The listing builds one solid part. Answer for the finished solid, in the listing's coordinates (mm). A direction names the side the tool comes from. Round coordinates to 2 decimals unless told otherwise and drop trailing zeros. Write each loop counter-clockwise with the first axis right and the second up, starting at its lowest first coordinate (ties: lowest second). Pieces come first, ordered by that corner, then holes.
Item 1: For a pull along X with two mould halves and no side action, classify faces 3 (the face through (-29.289, 4.196, 5.07)), 4 (the face through (-13, -6, 5)), 5 (the face through (-14.669, 0.526, 4.93)) as +X half, -X half, draft (parallel to the pull), parting line (faces both ways), or undercut.
Item 2: Find the intervals of material crossed by probe 1 along Y at (x, z) = (-13, 3); probe 2 along Z at (x, y) = (-6, -4); probe 3 along X at (y, z) = (0.5, 108.5), in increasing order.
Item 3: Each of these flat-tipped pins is pushed along its axis until it touches: pin 1 (6 mm diameter, centred on x = -13.5, y = 2, fed in from +Z); pin 2 (1 mm diameter, centred on x = -2.5, y = 2.5, fed in from -Z); pin 3 (5 mm diameter, centred on y = -4, z = 25, fed in from +X); pin 4 (5 mm diameter, centred on x = -21, z = 135, fed in from +Y). Where does it stop, or does it pass through?
Item 4: Find section A-A on x = -3. Give the vertices of the cut face in (y, z), then the cut area to 3 significant figures.
Item 5: A tool of negligible diameter and unlimited length cuts with its end or side. For faces 1 (the face through (-19, 0, 94)), 2 (the face through (-25, 0, 180)), from which of +Z, -Z, +X, -X, +Y, -Y can it reach the whole face along a straight path? Write none if from no direction.
Item 6: Find section D-D on z = 147.5. Give the vertices of the cut face in (x, y).
```python
from build123d import *

# Parameters (mm, degrees)
SKETCH1_W           = 36
SKETCH1_H           = 12
BOSS_EXTRUDE1_DEPTH = 10
SKETCH2_R           = 6
BOSS_EXTRUDE2_DEPTH = 170
CUT_EXTRUDE4_REACH  = 184.748
SKETCH7_R           = 1.75
FILLET1_R           = 6


with BuildPart() as part:
    # Sketch1 → Boss-Extrude1 (new body)
    with BuildSketch(Plane.XY):
        with Locations((-13, 0)):
            Rectangle(SKETCH1_W, SKETCH1_H)
    extrude(amount=BOSS_EXTRUDE1_DEPTH)

    # Sketch2 → Boss-Extrude2 (add)
    with BuildSketch(Plane.XY.offset(10)):
        with Locations(Location((-25, 0, 0), (0, 0, 180))):
            Circle(SKETCH2_R)
    extrude(amount=BOSS_EXTRUDE2_DEPTH)

    # Sketch7 → Cut-Extrude4 (cut, up to next)
    with BuildSketch(Plane(origin=(0, 0, 0), x_dir=(-1, 0, 0), z_dir=(0, 0, -1)), mode=Mode.PRIVATE) as cut_extrude4_sk1:
        with Locations((3, 0)):
            Circle(SKETCH7_R)
    cut_extrude4_tool1 = extrude(cut_extrude4_sk1.sketch, amount=-CUT_EXTRUDE4_REACH, mode=Mode.PRIVATE) & part.part
    # Sketch7 → Cut-Extrude4 (cut, up to next)
    with BuildSketch(Plane(origin=(0, 0, 0), x_dir=(-1, 0, 0), z_dir=(0, 0, -1)), mode=Mode.PRIVATE) as cut_extrude4_sk2:
        with Locations((13, 0)):
            Circle(SKETCH7_R)
    cut_extrude4_tool2 = extrude(cut_extrude4_sk2.sketch, amount=-CUT_EXTRUDE4_REACH, mode=Mode.PRIVATE) & part.part
    add(cut_extrude4_tool1.solids().sort_by_distance((-3, 0, 0))[0], mode=Mode.SUBTRACT)
    add(cut_extrude4_tool2.solids().sort_by_distance((-13, 0, 0))[0], mode=Mode.SUBTRACT)

    # Fillet1
    fillet1_edges = [part.edges().sort_by_distance(p)[0] for p in [
        (5, -6, 5),
        (5, 6, 5),
        (-31, -6, 5),
        (-31, 6, 5),
    ]]
    fillet(fillet1_edges, radius=FILLET1_R - 0.0001)  # a hair under: the kernel refuses the full size


solid = part.part
```
Check values:
1. face 3: -X half
1. face 4: draft
1. face 5: undercut
2. probe 1: y = -6 to -1.75, 1.75 to 6
2. probe 2: z = 0 to 10
2. probe 3: x = -30.98 to -19.02
3. pin 1: stops at z = 10
3. pin 2: stops at z = 0
3. pin 3: stops at x = -19.19
3. pin 4: stops at y = 5.81
4. outline: (-6, 0) - (-1.75, 0) - (-1.75, 10) - (-6, 10) - close; (1.75, 0) - (6, 0) - (6, 10) - (1.75, 10) - close
4. area: 85.0 mm2
5. face 1: +Z
5. face 2: +Z, +X, -X, +Y, -Y
6. outline: circle Ø12 at (-25, 0)
